For this review, take the finished solid that the model builds, in its own axes (mm). A direction names the side the tool comes from. Coordinates: 2 decimals unless noted, no trailing zeros. Order: outer loops, then holes, each group sorted by start corner. A loop starts at its lowest first (then second) coordinate and runs counter-clockwise, first axis right, second up.
from build123d import *

# Parameters (mm, degrees)
SKETCH_2_W          = 10
SKETCH_2_H          = 5
EXTRUDE_1_DEPTH     = 1.5
SKETCH_3_R          = 1.55
CUT_EXTRUDE_1_DEPTH = 1.5
SKETCH_4_W          = 5
SKETCH_4_H          = 5
EXTRUDE_2_DEPTH     = 61
SKETCH_5_W          = 10
SKETCH_5_H          = 5
EXTRUDE_3_DEPTH     = 1.5
SKETCH_6_R          = 1.55
CUT_EXTRUDE_2_DEPTH = 1.5
SKETCH_7_R          = 1.5
EXTRUDE_4_DEPTH     = 15
SKETCH_11_R         = 1.55
CUT_EXTRUDE_3_DEPTH = 10


with BuildPart() as part:
    # 草图2 → 凸台-拉伸1 (new body)
    with BuildSketch(Plane(origin=(0, 0, 0), x_dir=(1, 0, 0), z_dir=(0, 1, 0))):
        Rectangle(SKETCH_2_W, SKETCH_2_H)
    extrude(amount=EXTRUDE_1_DEPTH)

    # 草图3 → 切除-拉伸1 (cut)
    with BuildSketch(Plane.XZ):
        with Locations(Location((-2.5, 0, 0), (0, 0, 270))):
            Circle(SKETCH_3_R)
    extrude(amount=-CUT_EXTRUDE_1_DEPTH, mode=Mode.SUBTRACT)

    # 草图4 → 凸台-拉伸2 (add)
    with BuildSketch(Plane.XZ):
        with Locations((2.5, 0)):
            Rectangle(SKETCH_4_W, SKETCH_4_H)
    extrude(amount=EXTRUDE_2_DEPTH)

    # 草图5 → 凸台-拉伸3 (add)
    with BuildSketch(Plane.XZ.offset(61)):
        Rectangle(SKETCH_5_W, SKETCH_5_H)
    extrude(amount=EXTRUDE_3_DEPTH)

    # 草图6 → 切除-拉伸2 (cut)
    with BuildSketch(Plane.XZ.offset(62.5)):
        with Locations(Location((-2.5, 0, 0), (0, 0, 270))):
            Circle(SKETCH_6_R)
    extrude(amount=-CUT_EXTRUDE_2_DEPTH, mode=Mode.SUBTRACT)

    # 草图7 → 凸台-拉伸4 (add)
    with BuildSketch(Plane(origin=(0, 1.5, 0), x_dir=(1, 0, 0), z_dir=(0, 1, 0))):
        with Locations(Location((2.5, 0, 0), (0, 0, 270))):
            Circle(SKETCH_7_R)
    extrude(amount=EXTRUDE_4_DEPTH)

    # 草图11 → 切除-拉伸3 (cut)
    with BuildSketch(Plane.XZ.offset(62.5)):
        with Locations(Location((2.5, 0, 0), (0, 0, 270))):
            Circle(SKETCH_11_R)
    extrude(amount=-CUT_EXTRUDE_3_DEPTH, mode=Mode.SUBTRACT)


solid = part.part
1. Take a section at B-B, the plane x = -2.5. Give the boundary of the cut face in (y, z), plus the area to 3 significant figures.
Answer below:
outline: (-62.5, -2.5) - (-61, -2.5) - (-61, -1.55) - (-62.5, -1.55) - close; (-62.5, 1.55) - (-61, 1.55) - (-61, 2.5) - (-62.5, 2.5) - close; (0, -2.5) - (1.5, -2.5) - (1.5, -1.55) - (0, -1.55) - close; (0, 1.55) - (1.5, 1.55) - (1.5, 2.5) - (0, 2.5) - close
area: 5.70 mm2
2. Take a section at C-C, the plane y = -22. Give the boundary of the cut face in (x, z).
Answer below:
outline: (0, -2.5) - (5, -2.5) - (5, 2.5) - (0, 2.5) - close
3. Clearance check with flat-ended pins moving along their axes: pin 1 Ø2.5 at (x, z) = (-2, -0.5) entering from +Y; pin 2 Ø3 at (x, z) = (2.5, 0) entering from -Y. State where each tip first meets the part, or that it passes through.
Answer below:
pin 1: stops at y = 1.5
pin 2: stops at y = -52.5
4. To check wall thickness, follow L1, parallel to X at y = -61.85, z = 0; L2, parallel to X at y = 1, z = 0; L3, parallel to Y at x = 2.25, z = -2.15. State the ranges of each line that lie inside material, in increasing order.
Answer below:
L1: x = -5 to -4.05, -0.95 to 0.95, 4.05 to 5
L2: x = -5 to -4.05, -0.95 to 5
L3: y = -62.5 to 1.5
5. Take a section at D-D, the plane x = 1.75. Give the boundary of the cut face in (y, z), plus the area to 3 significant figures.
Answer below:
outline: (-62.5, -2.5) - (1.5, -2.5) - (1.5, -1.3) - (16.5, -1.3) - (16.5, 1.3) - (1.5, 1.3) - (1.5, 2.5) - (-62.5, 2.5) - (-62.5, 1.36) - (-52.5, 1.36) - (-52.5, -1.36) - (-62.5, -1.36) - close
area: 332 mm2
6. The part is to be moulded in two halves that separate along X. For faces 6 (the face through (-3.875, -61.76, -0.715)), 7 (the face through (3, 16.5, 0)), 8 (the face through (-5, -62, 0)), say which applies: +X half, -X half, draft (parallel to the pull), parting line (faces both ways), or undercut.
Answer below:
face 6: undercut
face 7: draft
face 8: -X half
7. Take a section at A-A, the plane z = 0. Give the boundary of the cut face in (x, y), plus the area to 3 significant figures.
Answer below:
outline: (-5, -62.5) - (-4.05, -62.5) - (-4.05, -61) - (-5, -61) - close; (-5, 0) - (-4.05, 0) - (-4.05, 1.5) - (-5, 1.5) - close; (-0.95, -62.5) - (0.95, -62.5) - (0.95, -52.5) - (4.05, -52.5) - (4.05, -62.5) - (5, -62.5) - (5, 1.5) - (4, 1.5) - (4, 16.5) - (1, 16.5) - (1, 1.5) - (-0.95, 1.5) - (-0.95, 0) - (0, 0) - (0, -61) - (-0.95, -61) - close
area: 340 mm2
8. Machinability: for faces 1 (the face through (0.987, -57.57, 0.336)), 2 (the face through (1, 9, 0)), 3 (the face through (5, -30, 0)), 4 (the face through (-3.875, 0.74, -0.715)), 5 (the face through (0, -30, 0)), which of the approach directions +Z, -Z, +X, -X, +Y, -Y give a long, thin tool a straight path to every point of the face, cutting with its end or side? Answer none if there is none.
Answer below:
face 1: -Y
face 2: +Y
face 3: +Z, -Z, +X, +Y, -Y
face 4: +Y, -Y
face 5: +Z, -Z, -X
